```python
from build123d import *

# Parameters (mm, degrees)
SKETCH_1_W          = 80
SKETCH_1_H          = 20
SKETCH_1_R          = 3
EXTRUDE_1_DEPTH     = 3
SKETCH_2_W          = 80
SKETCH_2_H          = 30
EXTRUDE_2_DEPTH     = 3
CUT_EXTRUDE_1_DEPTH = 20


with BuildPart() as part:
    # 草图1 → 凸台-拉伸1 (new body)
    with BuildSketch(Plane.XY):
        Rectangle(SKETCH_1_W, SKETCH_1_H)
        with Locations((20, 0)):
            Circle(SKETCH_1_R, mode=Mode.SUBTRACT)
        with Locations((-20, 0)):
            Circle(SKETCH_1_R, mode=Mode.SUBTRACT)
    extrude(amount=EXTRUDE_1_DEPTH)

    # 草图2 → 凸台-拉伸2 (add)
    with BuildSketch(Plane(origin=(0, 10, 0), x_dir=(1, 0, 0), z_dir=(0, 1, 0))):
        with Locations((0, -15)):
            Rectangle(SKETCH_2_W, SKETCH_2_H)
    extrude(amount=-EXTRUDE_2_DEPTH)

    # 草图3 → 切除-拉伸1 (cut)
    with BuildSketch(Plane(origin=(0, 10, 0), x_dir=(1, 0, 0), z_dir=(0, 1, 0))):
        with BuildLine():
            Line((-1.5, -4.5), (-1.5, -30))
            Line((-1.5, -30), (1.5, -30))
            Line((1.5, -30), (1.5, -4.5))
            ThreePointArc((1.5, -4.5), (0, -3), (-1.5, -4.5))
        make_face()
        with BuildLine():
            Line((33.5, -4.5), (33.5, -30))
            Line((33.5, -30), (36.5, -30))
            Line((36.5, -30), (36.5, -4.5))
            ThreePointArc((36.5, -4.5), (35, -3), (33.5, -4.5))
        make_face()
        with BuildLine():
            Line((-36.5, -4.5), (-36.5, -30))
            Line((-36.5, -30), (-33.5, -30))
            Line((-33.5, -30), (-33.5, -4.5))
            ThreePointArc((-33.5, -4.5), (-35, -3), (-36.5, -4.5))
        make_face()
    extrude(amount=-CUT_EXTRUDE_1_DEPTH, mode=Mode.SUBTRACT)


solid = part.part
```
Here's how the part is built. I have some questions about the finished solid (model axes, mm). A direction names the side the tool comes from. Give positions to 0.01 mm unless a question says otherwise; leave off trailing zeros. Loops run counter-clockwise (first coordinate to the right, second up) from the corner with the lowest first, then second, coordinate; pieces in that order, holes last. Notation, with made-up numbers: M -39.75,17.25 L -23.75,17.25 A20 cw -23.75,26.25 Z; hole C -3.5,9.25 d7. An arc over 180 degrees is marked long. Return JSON: item names as keys, results as strings.
Item 1: Imagine slicing it at D-D on x = 13. List the corners of the cut face in (y, z) for me, then the cut area to 3 significant figures.
A:
{"outline": "M -10,0 L 10,0 L 10,30 L 7,30 L 7,3 L -10,3 Z", "area": "141 mm^2"}
Item 2: I'm going to push flat-ended pins straight in: pin 1 Ø3 at (x, z) = (-20, 10.5) entering from -Y; pin 2 Ø8 at (x, y) = (20, 0) entering from +Z. Where does each tip first touch, or does it pass through?
A:
{"pin 1": "stops at y = 7", "pin 2": "stops at z = 3"}
Item 3: Imagine slicing it at B-B on y = 0. List the corners of the cut face in (x, z) for me.
A:
{"outline": "M -40,0 L -23,0 L -23,3 L -40,3 Z; M -17,0 L 17,0 L 17,3 L -17,3 Z; M 23,0 L 40,0 L 40,3 L 23,3 Z"}
Item 4: Imagine slicing it at C-C on x = -20. List the corners of the cut face in (y, z) for me.
A:
{"outline": "M -10,0 L -3,0 L -3,3 L -10,3 Z; M 3,0 L 10,0 L 10,30 L 7,30 L 7,3 L 3,3 Z"}
Item 5: On a 3-axis mill with a long thin cutter (end or side, diameter ignored), from which of +Z, -Z, +X, -X, +Y, -Y can I reach the whole of each face in a straight line? I mean faces 4 (the cylindrical face through (17, 0, 1)), 5 (the flat face through (-18, 7, 16)), 6 (the flat face through (1.5, 9, 17)). Say none if no direction works.
A:
{"face 4": "+Z, -Z", "face 5": "+Z, +X, -X, -Y", "face 6": "+Z, +Y, -Y"}
Item 6: Please list where these lines run through material, in increasing order: line 1 (Y direction, x = -20, z = 1.7); line 2 (Z direction, x = -3, y = -5.5); line 3 (Y direction, x = 30, z = 19.5).
A:
{"line 1": "y = -10 to -3, 3 to 10", "line 2": "z = 0 to 3", "line 3": "y = 7 to 10"}
Item 7: Imagine slicing it at A-A on z = 23.25. List the corners of the cut face in (x, y) for me.
A:
{"outline": "M -40,7 L -36.5,7 L -36.5,10 L -40,10 Z; M -33.5,7 L -1.5,7 L -1.5,10 L -33.5,10 Z; M 1.5,7 L 33.5,7 L 33.5,10 L 1.5,10 Z; M 36.5,7 L 40,7 L 40,10 L 36.5,10 Z"}
Item 8: Thinking about a two-plate mould opening in X: for faces 1 (the flat face through (40, 8, 10)), 2 (the flat face through (-1, 0, 0)), 3 (the flat face through (-33.5, 9, 17)), which applies, released by +X, released by -X, zero draft, split by the parting line, or undercut?
A:
{"face 1": "released by +X", "face 2": "zero draft", "face 3": "undercut"}
